```python
from build123d import *

# Parameters (mm, degrees)
F1_DEPTH = 24
F2_T     = -1.5
F3_R     = 5
F4_DEPTH = 5


with BuildPart() as f1:
    # F0 (on Front) → F1 (new body)
    with BuildSketch(Plane.XZ):
        with BuildLine():
            Line((0, 42), (0, 0))
            Line((0, 0), (30, 0))
            Line((30, 0), (30, 12))
            Line((30, 12), (22, 12))
            Line((22, 12), (22, 32))
            ThreePointArc((22, 32), (18.7650208971, 54.0830459736), (0, 42))
        make_face()
    extrude(amount=F1_DEPTH)

    # F2
    f2_openings = [f1.faces().sort_by_distance(p)[0] for p in [
        (15, -12, 0),
    ]]
    offset(amount=F2_T, openings=f2_openings, kind=Kind.INTERSECTION)

    # F3 (on face) → F4 (cut)
    with BuildSketch(Plane(origin=(0, 0, 0), x_dir=(-1, 0, 0), z_dir=(0, 1, 0))):
        with Locations((-13.2727272727, 42)):
            Circle(F3_R)
    extrude(amount=-F4_DEPTH, mode=Mode.SUBTRACT)


solid = f1.part
```
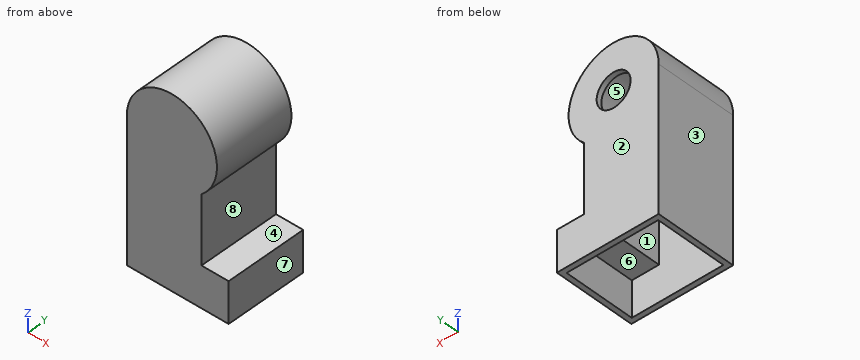
For this review, take the finished solid that the model builds, in its own axes (mm). Face numbers are marked on the shaded views. A direction names the side the tool comes from. Round coordinates to 2 decimals unless told otherwise and drop trailing zeros. Write each loop counter-clockwise with the first axis right and the second up, starting at its lowest first coordinate (ties: lowest second). Pieces come first, ordered by that corner, then holes. Notation, with made-up numbers: M 79,-17 L 109,-17 A31 ccw 109,18 Z; hole C 59.5,-16.75 d9. An arc over 180 degrees is marked long. One line per item, written item: value. Start each with the question number.
(1) Wall thickness on line 1 (X direction, y = -16.5, z = 16.5); line 2 (Y direction, x = 10.75, z = 22); line 3 (Z direction, x = 27, y = -21): over which ranges is each line inside the solid? List them lowest first.
(2) We need section C-C (x = 13.5). Give the boundary of the cut face in (y, z).
(3) The part is to be moulded in two halves that separate along Z. For the marked faces 6, 7 and 8, say which applies: released by +Z, released by -Z, zero draft, split by the parting line, or undercut.
(4) Insertion check: pin 1 (6.5 mm diameter, centred on x = 27, y = -15, fed in from +Z); pin 2 (6.5 mm diameter, centred on x = 24, y = -8, fed in from -Z); pin 3 (2 mm diameter, centred on x = 15, y = -14.5, fed in from +Z). Each pin has a flat end and moves straight along its axis. Give the tip position at first contact, or say it passes through.
(5) We need section D-D (z = 17.5). Give the boundary of the cut face in (x, y), and give its area (3 significant figures).
(6) We need section A-A (z = 8.5). Give the boundary of the cut face in (x, y), and give its area (3 significant figures).
(7) We need section B-B (y = -2.25). Give the boundary of the cut face in (x, z).
(8) Machinability: for the marked faces 1, 2, 3, 4 and 5, which of the approach directions +Z, -Z, +X, -X, +Y, -Y give a long, thin tool a straight path to every point of the face, cutting with its end or side? Answer none if there is none.
Result:
1. line 1: 0 to 1.5, 20.5 to 22
1. line 2: -24 to -22.5, -1.5 to 0
1. line 3: 10.5 to 12
2. outline: M -24,0 L -22.5,0 L -22.5,53.77 L -1.5,53.77 L -1.5,46.99 L 0,46.99 L 0,55.27 L -24,55.27 Z; M -1.5,0 L 0,0 L 0,37.01 L -1.5,37.01 Z
3. face 6: released by -Z
3. face 7: zero draft
3. face 8: undercut
4. pin 1: z = 50.15
4. pin 2: z = 10.5
4. pin 3: z = 55.25
5. outline: M 0,-24 L 22,-24 L 22,0 L 0,0 Z; hole M 1.5,-22.5 L 20.5,-22.5 L 20.5,-1.5 L 1.5,-1.5 Z
5. area: 129 mm²
6. outline: M 0,-24 L 30,-24 L 30,0 L 0,0 Z; hole M 1.5,-22.5 L 28.5,-22.5 L 28.5,-1.5 L 1.5,-1.5 Z
6. area: 153 mm²
7. outline: M 0,0 L 1.5,0 L 1.5,42 A11.77 cw long 20.5,32.71 L 20.5,10.5 L 28.5,10.5 L 28.5,0 L 30,0 L 30,12 L 22,12 L 22,32 A13.27 ccw long 0,42 Z
8. face 1: -Z
8. face 2: +Z, -Z, +X, -X, +Y
8. face 3: +Z, -Z, -X, +Y, -Y
8. face 4: +X, +Y, -Y
8. face 5: none
